```python
from build123d import *

# Parameters (mm, degrees)
BOSS_EXTRUDE1_DEPTH = 10
SKETCH2_R           = 2.85
CUT_EXTRUDE1_DEPTH  = 3
SKETCH3_R           = 2
CUT_EXTRUDE2_DEPTH  = 65.517439503
SKETCH4_R           = 8
CUT_EXTRUDE5_DEPTH  = 5
SKETCH6_R           = 3.5
CUT_EXTRUDE6_DEPTH  = 65.517439503
CUT_EXTRUDE7_DEPTH  = 65.517439503


with BuildPart() as part:
    # Sketch1 → Boss-Extrude1 (new body)
    with BuildSketch(Plane(origin=(0, 0, 0), x_dir=(1, 0, 0), z_dir=(0, 1, 0))):
        with BuildLine():
            Line((-12.5, 0), (-12.5, 50))
            ThreePointArc((-12.5, 50), (0, 62.5), (12.5, 50))
            Line((12.5, 50), (12.5, 0))
            ThreePointArc((12.5, 0), (0, -12.5), (-12.5, 0))
        make_face()
    extrude(amount=BOSS_EXTRUDE1_DEPTH)

    # Sketch2 → Cut-Extrude1 (cut)
    with BuildSketch(Plane(origin=(0, 10, 0), x_dir=(1, 0, 0), z_dir=(0, 1, 0))):
        with Locations(Location((0, 9, 0), (0, 0, 270))):
            Circle(SKETCH2_R)
        with Locations(Location((9, 0, 0), (0, 0, 270))):
            Circle(SKETCH2_R)
        with Locations(Location((0, -9, 0), (0, 0, 270))):
            Circle(SKETCH2_R)
        with Locations(Location((-9, 0, 0), (0, 0, 270))):
            Circle(SKETCH2_R)
    extrude(amount=-CUT_EXTRUDE1_DEPTH, mode=Mode.SUBTRACT)

    # Sketch3 → Cut-Extrude2 (cut, through all)
    with BuildSketch(Plane(origin=(0, 10, 0), x_dir=(1, 0, 0), z_dir=(0, 1, 0))):
        with Locations(Location((0, 9, 0), (0, 0, 270))):
            Circle(SKETCH3_R)
        with Locations(Location((9, 0, 0), (0, 0, 270))):
            Circle(SKETCH3_R)
        with Locations(Location((0, -9, 0), (0, 0, 270))):
            Circle(SKETCH3_R)
        with Locations(Location((-9, 0, 0), (0, 0, 270))):
            Circle(SKETCH3_R)
    extrude(amount=-CUT_EXTRUDE2_DEPTH, mode=Mode.SUBTRACT)

    # Sketch4 → Cut-Extrude5 (cut)
    with BuildSketch(Plane.XZ.offset(-10)):
        with Locations(Location((0, -50, 0), (0, 0, 270))):
            Circle(SKETCH4_R)
    extrude(amount=CUT_EXTRUDE5_DEPTH, mode=Mode.SUBTRACT)

    # Sketch6 → Cut-Extrude6 (cut, through all)
    with BuildSketch(Plane(origin=(0, 10, 0), x_dir=(1, 0, 0), z_dir=(0, 1, 0))):
        with Locations(Location((0, 50, 0), (0, 0, 270))):
            Circle(SKETCH6_R)
    extrude(amount=-CUT_EXTRUDE6_DEPTH, mode=Mode.SUBTRACT)

    # Sketch7 → Cut-Extrude7 (cut, through all)
    with BuildSketch(Plane.XZ):
        Polygon((4.618802154, -50), (2.309401077, -46), (-2.309401077, -46), (-4.618802154, -50), (-2.309401077, -54), (2.309401077, -54), align=None)
    extrude(amount=-CUT_EXTRUDE7_DEPTH, mode=Mode.SUBTRACT)


solid = part.part
```
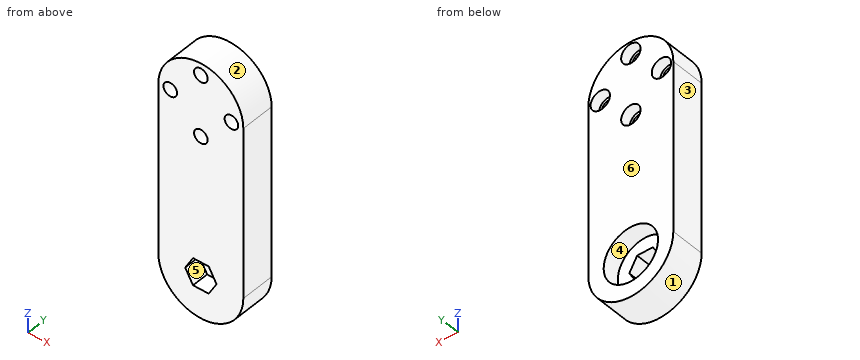
Check sheet for the modelled part. Datum: model origin and axes. Units: mm. Face numbers are marked on the shaded views. A direction names the side the tool comes from. Give positions to 0.01 mm unless a question says otherwise; leave off trailing zeros. Order: outer loops, then holes, each group sorted by start corner. A loop starts at its lowest first (then second) coordinate and runs counter-clockwise, first axis right, second up. Notation, with made-up numbers: (75, -18.75) -> (93, -18.75) arc R20 ccw to (93, 1.25) -> close; hole circle Ø9 at (-24.5, -2). An arc over 180 degrees is marked (long way). Use CSV: the item, a comma, the result in double quotes. Start each with the question number.
1) Material ranges on line 1 (Z direction, x = 1.75, y = 6.5); line 2 (Z direction, x = -7, y = 7.75); line 3 (Z direction, x = -1.75, y = 1.5), recorded low to high. Write a range as from..to.
2) Sectioned sample at D-D, the plane z = 1. Record the boundary of the cut face in (x, y), plus the area to 3 significant figures.
3) Mould release check, pull along Z, two halves, no side actions. Record for the marked faces 1, 2, 3 and 4: released by +Z, released by -Z, zero draft, split by the parting line, or undercut.
4) Sectioned sample at B-B, the plane x = 0. Record the boundary of the cut face in (y, z), plus the area to 3 significant figures.
5) Go/stop test with flat-tipped pins: P1, Ø6.5, axis at x = 7.5, z = -1, coming from the +Y side; P2, Ø5, axis at x = 0, z = 9, coming from the +Y side; P3, Ø6, axis at x = -6.5, y = 4, coming from the +Z side; P4, Ø5, axis at x = -1.5, z = -51, coming from the +Y side. Record where each tip stops, or that it passes through.
6) Set-up check for the marked faces 5 and 6: record each of +Z, -Z, +X, -X, +Y, -Y from which the full face is reachable in a straight line by a thin tool's end or side.
7) Sectioned sample at A-A, the plane z = -9. Record the boundary of the cut face in (x, y), plus the area to 3 significant figures.
8) Sectioned sample at C-C, the plane y = 8.5. Record the boundary of the cut face in (x, z), plus the area to 3 significant figures.
Recorded:
1,line 1,"-62.38..-57.81, -42.19..-9.97, -8.03..8.03, 9.97..12.38"
1,line 2,"-60.36..-53.87, -46.13..-2.03, 2.03..10.36"
1,line 3,"-62.38..-54, -46..-9.97, -8.03..8.03, 9.97..12.38"
2,outline,"(-12.46, 0) -> (-10.73, 0) -> (-10.73, 7) -> (-11.67, 7) -> (-11.67, 10) -> (-12.46, 10) -> close; (-7.27, 0) -> (7.27, 0) -> (7.27, 7) -> (6.33, 7) -> (6.33, 10) -> (-6.33, 10) -> (-6.33, 7) -> (-7.27, 7) -> close; (10.73, 0) -> (12.46, 0) -> (12.46, 10) -> (11.67, 10) -> (11.67, 7) -> (10.73, 7) -> close"
2,area,"169 mm2"
3,face 1,"released by -Z"
3,face 2,"released by +Z"
3,face 3,"zero draft"
3,face 4,"undercut"
4,outline,"(0, -62.5) -> (10, -62.5) -> (10, -58) -> (5, -58) -> (5, -54) -> (0, -54) -> close; (0, -46) -> (5, -46) -> (5, -42) -> (10, -42) -> (10, -11.85) -> (7, -11.85) -> (7, -11) -> (0, -11) -> close; (0, -7) -> (7, -7) -> (7, -6.15) -> (10, -6.15) -> (10, 6.15) -> (7, 6.15) -> (7, 7) -> (0, 7) -> close; (0, 11) -> (7, 11) -> (7, 11.85) -> (10, 11.85) -> (10, 12.5) -> (0, 12.5) -> close"
4,area,"540 mm2"
5,P1,"y = 10"
5,P2,"y = 7"
5,P3,"z = 12"
5,P4,"y = 5"
6,face 5,"+Y, -Y"
6,face 6,"+Z, -Z, +X, -X, +Y"
7,outline,"(-12.5, 0) -> (-2, 0) -> (-2, 7) -> (-2.85, 7) -> (-2.85, 10) -> (-12.5, 10) -> close; (2, 0) -> (12.5, 0) -> (12.5, 10) -> (2.85, 10) -> (2.85, 7) -> (2, 7) -> close"
7,area,"205 mm2"
8,outline,"(-12.5, -50) arc R12.5 ccw to (12.5, -50) -> (12.5, 0) arc R12.5 ccw to (-12.5, 0) -> close; hole circle Ø5.7 at (-9, 0); hole circle Ø16 at (0, -50); hole circle Ø5.7 at (0, -9); hole circle Ø5.7 at (0, 9); hole circle Ø5.7 at (9, 0)"
8,area,"1,440 mm2"
